Design review of the part shown in the three views and the two pictorial views. Dimensions are in mm from the part's minimum x, y and z. Round coordinates to 2 decimals unless told otherwise and drop trailing zeros. Order: outer loops, then holes, each group sorted by start corner. A loop starts at its lowest first (then second) coordinate and runs counter-clockwise, first axis right, second up.
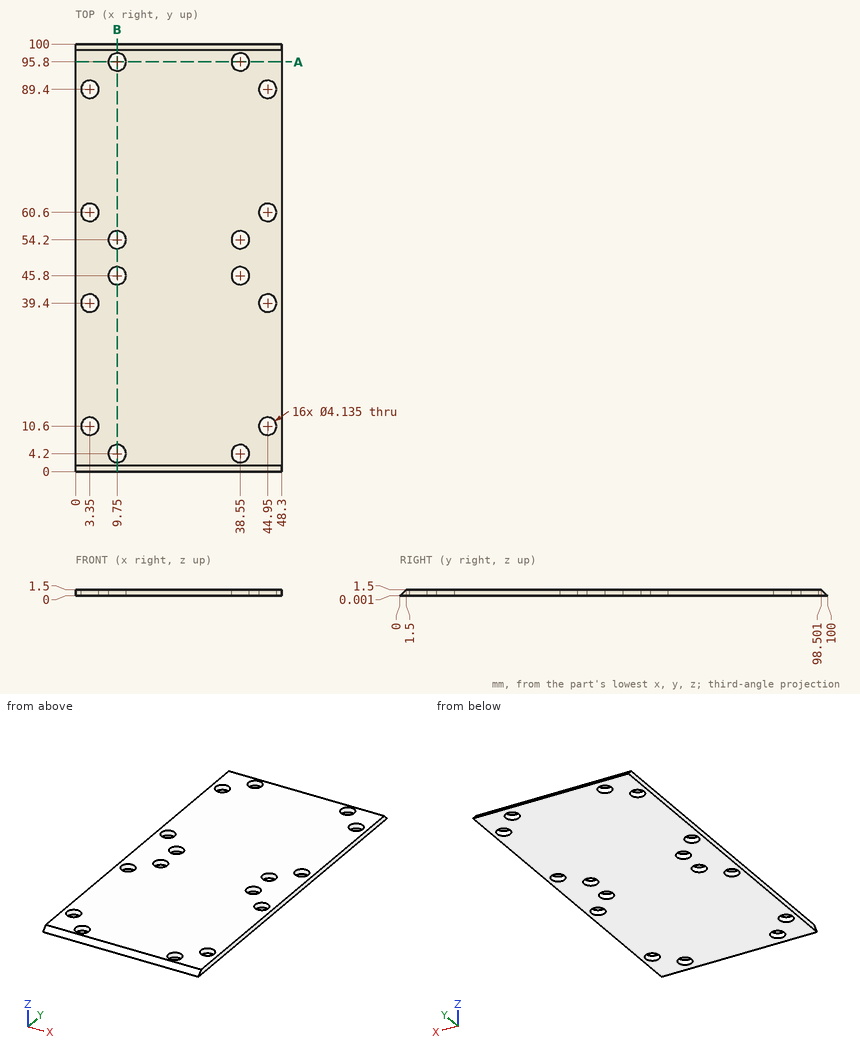
1) Take a section at B-B on x = 9.75. State how many separate pieces and enclosed holes the cut face has, plus the area to 3 significant figures.
Results:
separate pieces: 5
enclosed holes: 0
area: 123 mm2
2) To check wall thickness, follow line 1 along X through (y, z) = (95.5, 0.15) (1 decimal); line 2 along X through (y, z) = (40.5, 1.1); line 3 along Y through (x, z) = (9, 1.4) (1 decimal). State the ranges of each line that lie inside material, in increasing order.
Results:
line 1: x = 0 to 7.7, 11.8 to 36.5, 40.6 to 48.3
line 2: x = 0 to 1.6, 5.1 to 43.2, 46.7 to 48.3
line 3: y = 1.4 to 2.3, 6.1 to 43.9, 47.7 to 52.3, 56.1 to 93.9, 97.7 to 98.6
3) Take a section at A-A on y = 95.8. Give the boundary of the cut face in (x, z).
Results:
outline: (0, 0) - (7.68, 0) - (7.68, 1.5) - (0, 1.5) - close; (11.82, 0) - (36.48, 0) - (36.48, 1.5) - (11.82, 1.5) - close; (40.62, 0) - (48.3, 0) - (48.3, 1.5) - (40.62, 1.5) - close
4) Clearance check with flat-ended pins moving along their axes: P1, Ø2.5, axis at x = 38.55, y = 95.8, coming from the +Z side; P2, Ø5.5, axis at x = 38.55, y = 45.8, coming from the -Z side. State where each tip first meets the part, or that it passes through.
Results:
P1: passes through
P2: stops at z = 0
